Geometry check sheet. Reference: the model listing, model coordinates, mm. Face numbers are marked on the shaded views. A direction names the side the tool comes from. Give positions to 0.01 mm unless a question says otherwise; leave off trailing zeros. Write each loop counter-clockwise with the first axis right and the second up, starting at its lowest first coordinate (ties: lowest second). Pieces come first, ordered by that corner, then holes. Notation, with made-up numbers: (-8.5, 67) - (7.5, 67) arc R18 ccw to (7.5, 77) - close; hole circle Ø2 at (-6.75, 58). An arc over 180 degrees is marked (long way). Use a Markdown table: item, result.
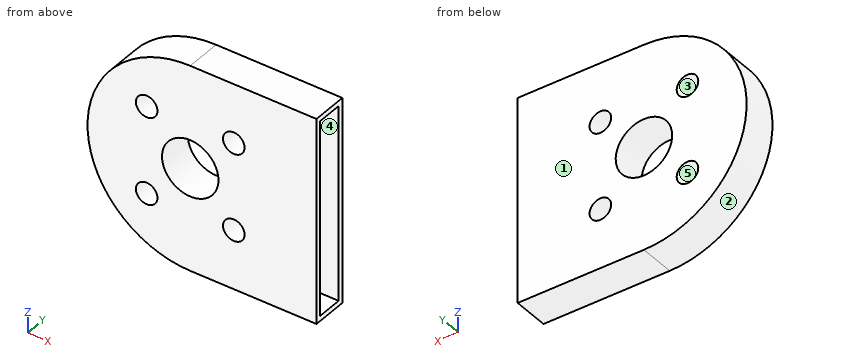
```python
from build123d import *

# Parameters (mm, degrees)
SKETCH1_R           = 10
SKETCH1_R_2         = 1.05
SKETCH1_R_3         = 2.75
BOSS_EXTRUDE1_DEPTH = 3.5
SKETCH8_R           = 1.05
CUT_EXTRUDE2_DEPTH  = 10
BOSS_EXTRUDE5_DEPTH = 3.5
SHELL2_T            = -0.5


with BuildPart() as part:
    # Sketch1 → Boss-Extrude1 (new body)
    with BuildSketch(Plane(origin=(0, 0, 0), x_dir=(1, 0, 0), z_dir=(0, 1, 0))):
        with Locations(Location((0, 0, 0), (0, 0, 270))):
            Circle(SKETCH1_R)
        with Locations(Location((-4.24264069, 4.24264069, 0), (0, 0, 270))):
            Circle(SKETCH1_R_2, mode=Mode.SUBTRACT)
        with Locations(Location((0, 0, 0), (0, 0, 270))):
            Circle(SKETCH1_R_3, mode=Mode.SUBTRACT)
    extrude(amount=BOSS_EXTRUDE1_DEPTH)

    # Sketch8 → Cut-Extrude2 (cut)
    with BuildSketch(Plane(origin=(0, 3.5, 0), x_dir=(1, 0, 0), z_dir=(0, 1, 0))):
        with Locations(Location((-4.24264069, -4.24264069, 0), (0, 0, 270))):
            Circle(SKETCH8_R)
        with Locations(Location((4.24264069, 4.24264069, 0), (0, 0, 270))):
            Circle(SKETCH8_R)
        with Locations(Location((4.24264069, -4.24264069, 0), (0, 0, 270))):
            Circle(SKETCH8_R)
    extrude(amount=-CUT_EXTRUDE2_DEPTH, mode=Mode.SUBTRACT)

    # Sketch11 → Boss-Extrude5 (add)
    with BuildSketch(Plane.XZ):
        with BuildLine():
            Line((12.293904652, 10), (0, 10))
            ThreePointArc((0, 10), (7.071067812, 7.071067812), (10, 0))
            ThreePointArc((10, 0), (7.071067812, -7.071067812), (0, -10))
            Line((0, -10), (12.293904652, -10))
            Line((12.293904652, -10), (12.293904652, 10))
        make_face()
    extrude(amount=-BOSS_EXTRUDE5_DEPTH)

    # Shell2
    shell2_openings = [part.faces().sort_by_distance(p)[0] for p in [
        (12.293904652, 1.75, 0),
    ]]
    offset(amount=SHELL2_T, openings=shell2_openings, kind=Kind.INTERSECTION)


solid = part.part
```
1) Section check A-A on z = 0. Record the boundary of the cut face in (x, y), then the cut area to 3 significant figures.
Working result:
| item | result |
|---|---|
| outline | (-10, 0) - (-2.75, 0) - (-2.75, 3.5) - (-10, 3.5) - close; (2.75, 0) - (12.29, 0) - (12.29, 0.5) - (3.25, 0.5) - (3.25, 3) - (12.29, 3) - (12.29, 3.5) - (2.75, 3.5) - close; hole (-9.5, 0.5) - (-3.25, 0.5) - (-3.25, 3) - (-9.5, 3) - close |
| area | 20.5 mm² |
2) Depth check by flat-ended pin: P1, Ø1.7, axis at x = -4.24, z = 4.24, coming from the +Y side. Enter the tip coordinate at first touch or a pass-through.
Working result:
| item | result |
|---|---|
| P1 | passes through |
3) Mould release check, pull along X, two halves, no side actions. Record for the marked faces 1, 2 and 3: pulls with the +X half, pulls with the -X half, needs draft (parallel to the pull), parting line crosses it, or undercut.
Working result:
| item | result |
|---|---|
| face 1 | needs draft |
| face 2 | pulls with the -X half |
| face 3 | undercut |
4) Section check B-B on x = -1.75. Record the boundary of the cut face in (y, z), then the cut area to 3 significant figures.
Working result:
| item | result |
|---|---|
| outline | (0, -9.85) - (3.5, -9.85) - (3.5, -2.12) - (0, -2.12) - close; (0, 2.12) - (3.5, 2.12) - (3.5, 9.85) - (0, 9.85) - close; hole (0.5, -9.34) - (3, -9.34) - (3, -2.74) - (0.5, -2.74) - close; hole (0.5, 2.74) - (3, 2.74) - (3, 9.34) - (0.5, 9.34) - close |
| area | 21.1 mm² |
5) Material ranges on L1, parallel to X at y = 2, z = 0; L2, parallel to X at y = 1.95, z = -1.5; L3, parallel to Y at x = 5.5, z = -5.5, recorded low to high. Write a range as from..to.
Working result:
| item | result |
|---|---|
| L1 | x = -10..-9.5, -3.25..-2.75, 2.75..3.25 |
| L2 | x = -9.89..-9.38, -2.88..-2.3, 2.3..2.88 |
| L3 | y = 0..0.5, 3..3.5 |
6) Set-up check for the marked faces 4 and 5: record each of +Z, -Z, +X, -X, +Y, -Y from which the full face is reachable in a straight line by a thin tool's end or side.
Working result:
| item | result |
|---|---|
| face 4 | none |
| face 5 | +Y, -Y |
7) Section check D-D on x = -6.75. Record the boundary of the cut face in (y, z).
Working result:
| item | result |
|---|---|
| outline | (0, -7.38) - (3.5, -7.38) - (3.5, 7.38) - (0, 7.38) - close; hole (0.5, -6.68) - (3, -6.68) - (3, 6.68) - (0.5, 6.68) - close |
8) Section check C-C on y = 1.05. Count the separate pieces of the cut face and the enclosed holes in it, then the cut area to 3 significant figures.
Working result:
| item | result |
|---|---|
| separate pieces | 6 |
| enclosed holes | 5 |
| area | 53.4 mm² |
